Check sheet for the modelled part. Datum: model origin and axes. Units: mm. A direction names the side the tool comes from. Round coordinates to 2 decimals unless told otherwise and drop trailing zeros. Loops run counter-clockwise (first coordinate to the right, second up) from the corner with the lowest first, then second, coordinate; pieces in that order, holes last. Notation, with made-up numbers: M 44.25,34.5 L 98.25,34.5 A18 cw 98.25,58.5 Z; hole C 55,15 d1. An arc over 180 degrees is marked long. Write item = value, one per line. Start each with the question number.
(1) Scan lines: L1, parallel to Y at x = -24, z = 10; L2, parallel to X at y = -6.5, z = 25; L3, parallel to X at y = -1.75, z = 74.5. Record each from-to range of solid material in increasing order. Write a range as from..to.
(2) Cross-section at C-C on y = -13.75. Record the boundary of the cut face in (x, z).
(3) Go/stop test with a flat-tipped pin: P1, Ø7.5, axis at y = -8.5, z = 35.5, coming from the +X side. Record where the tip stops, or that it passes through.
(4) Set-up check for faces 1 (the face through (2, -25.5, 39)), 2 (the face through (2, -1.5, 39)): record each of +Z, -Z, +X, -X, +Y, -Y from which the full face is reachable in a straight line by a thin tool's end or side.
(5) Mould release check, pull along Y, two halves, no side actions. Record for faces 3 (the face through (-1, -23, 0)), 4 (the face through (-108.196, -23.789, 40.56)), 5 (the face through (4, -22.5, 39)), 6 (the face through (4, 1.5, 39)): pulls with the +Y half, pulls with the -Y half, needs draft (parallel to the pull), parting line crosses it, or undercut.
(6) Cross-section at B-B on z = 29.5. Record the boundary of the cut face in (x, y).
(7) Cross-section at A-A on x = -25.5. Record the boundary of the cut face in (y, z), plus the area to 3 significant figures.
from build123d import *

# Parameters (mm, degrees)
F0_W     = 3
F0_H     = 21
F1_DEPTH = 80
F2_R     = 3
F3_R     = 6


with BuildPart() as f1:
    # F0 (on Top) → F1 (new body)
    with BuildSketch(Plane.XY):
        Polygon((-110, 1.5), (-110, -1.5), (-107, -1.5), (110, -1.5), (110, 1.5), align=None)
        with Locations((-108.5, -12)):
            Rectangle(F0_W, F0_H)
        Polygon((-107, -22.5), (-110, -22.5), (-110, -25.5), (110, -25.5), (110, -22.5), align=None)
    extrude(amount=F1_DEPTH)

    # F2
    f2_edges = [f1.edges().sort_by_distance(p)[0] for p in [
        (-107, -1.5, 40),
        (-107, -22.5, 40),
    ]]
    fillet(f2_edges, radius=F2_R)

    # F3
    f3_edges = [f1.edges().sort_by_distance(p)[0] for p in [
        (-110, -25.5, 40),
        (-110, 1.5, 40),
    ]]
    fillet(f3_edges, radius=F3_R)


solid = f1.part
Result:
q1.L1 = -25.5..-22.5, -1.5..1.5
q1.L2 = -110..-107
q1.L3 = -109.33..-105.2
q2.outline = M -110,0 L -107,0 L -107,80 L -110,80 Z
q3.P1 = -107
q4.face_1 = +Z, -Z, +X, -X, -Y
q4.face_2 = +Z, -Z, +X
q5.face_3 = needs draft
q5.face_4 = pulls with the -Y half
q5.face_5 = undercut
q5.face_6 = pulls with the +Y half
q6.outline = M -110,-19.5 A6 ccw -104,-25.5 L 110,-25.5 L 110,-22.5 L -104,-22.5 A3 cw -107,-19.5 L -107,-4.5 A3 cw -104,-1.5 L 110,-1.5 L 110,1.5 L -104,1.5 A6 ccw -110,-4.5 Z
q7.outline = M -25.5,0 L -22.5,0 L -22.5,80 L -25.5,80 Z; M -1.5,0 L 1.5,0 L 1.5,80 L -1.5,80 Z
q7.area = 480 mm^2
